For this review, take the finished solid that the model builds, in its own axes (mm). A direction names the side the tool comes from. Give positions to 0.01 mm unless a question says otherwise; leave off trailing zeros. Loops run counter-clockwise (first coordinate to the right, second up) from the corner with the lowest first, then second, coordinate; pieces in that order, holes last. Notation, with made-up numbers: (19.5, 31) - (33.5, 31) arc R8 cw to (33.5, 42) - close; hole circle Ø8 at (6.5, -31). An arc over 180 degrees is marked (long way). Answer in a Markdown table with one row per item.
Autodesk Inventor part; units mm, degrees
ref_plane "YZ Plane" through (0, 0, 0) normal (1, 0, 0) x (0, 1, 0)
ref_plane "XZ Plane" through (0, 0, 0) normal (0, 1, 0) x (-1, 0, 0)
ref_plane "XY Plane" through (0, 0, 0) normal (0, 0, 1) x (1, 0, 0)
sketch "Sketch1" plane through (0, 0, 0) normal (0, 0, 1) x (1, 0, 0)
  line L0 (17, 4.5) -> (17, -4.5)
  line L1 (-17, -4.5) -> (-17, 4.5)
  arc A0 (-8.3666, -4.5) -> (8.3666, -4.5) centre (0, 0) ccw
  arc A1 (8.3666, 4.5) -> (-8.3666, 4.5) centre (0, 0) ccw
  line L2 (-17, 4.5) -> (-8.3666, 4.5)
  line L3 (8.3666, 4.5) -> (17, 4.5)
  line L4 (17, -4.5) -> (8.3666, -4.5)
  line L5 (-8.3666, -4.5) -> (-17, -4.5)
  line L6 (-17, 4.5) -> (17, -4.5) construction
  line L7 (-17, -4.5) -> (17, 4.5) construction
  point P0 (0, 0)
  point P1 (0, 0)
  dimension "d0" = 9
  dimension "d1" = 34
  dimension "d2" = 9.5
  dimension "d3" = 9
  dimension "d4" = 9.5
  dimension "d12" = 4.5
extrude "Extrusion1" add sketch "Sketch1" along normal blind 7
sketch "Sketch2" plane through (17, -4.5, 0) normal (1, 0, 0) x (0, 0, -1)
  arc A0 (-11.5, 9) -> (-11.5, 0) centre (-11.5, 4.5) ccw
  circle A1 centre (-11.5, 4.5) radius 2.25
  line L0 (-7, 9) -> (-11.5, 9)
  line L1 (-11.5, 0) -> (-7, 0)
  line L2 (-7, 0) -> (-7, 9)
  point P0 (0, 4.5)
  point P1 (-7, 0)
  dimension "d7" = 9
  dimension "d8" = 4.5
  dimension "d9" = 9
extrude "Extrusion2" add sketch "Sketch2" against normal blind 4.3
extrude "Extrusion3" add sketch "Sketch2" along normal blind 4.3 from surface at -34
sketch "Sketch3" plane through (-17, -4.5, 0) normal (0, -1, 0) x (1, 0, 0)
  line L0 (0, 6) -> (0, 0)
  line L1 (0, 0) -> (5, 0)
  line L2 (5, 0) -> (0, 6)
  line L3 (29, 0) -> (34, 0)
  line L4 (34, 0) -> (34, 6)
  line L5 (34, 6) -> (29, 0)
  point P0 (17, 0)
  dimension "d15" = 6
  dimension "d16" = 5
  dimension "d17" = 6
  dimension "d18" = 5
extrude "Extrusion4" cut sketch "Sketch3" against normal up to next
sketch "Sketch4" plane through (0, 0, 0) normal (0, 0, -1) x (-1, 0, 0)
  circle A0 centre (0, 0) radius 7.5
  dimension "d21" = 15
extrude "Extrusion5" add sketch "Sketch4" along normal blind 2.5
sketch "Sketch5" plane through (0, 0, 7) normal (0, 0, 1) x (1, 0, 0)
  circle A0 centre (0, 0) radius 7.5
  dimension "d24" = 15
extrude "Extrusion6" cut sketch "Sketch5" against normal blind 4
sketch "Sketch6" plane through (0, 0, -2.5) normal (0, 0, -1) x (-1, 0, 0)
  circle A0 centre (0, 0) radius 5.5
  dimension "d27" = 11
extrude "Extrusion7" cut sketch "Sketch6" against normal blind 4
sketch "Sketch7" plane through (0, 0, 1.5) normal (0, 0, -1) x (-1, 0, 0)
  circle A0 centre (0, 0) radius 5
  dimension "d30" = 10
extrude "Extrusion8" cut sketch "Sketch7" against normal up to next
sketch "Sketch9" plane through (0, 0, 0) normal (1, 0, 0) x (0, 1, 0)
  line L0 (-9.5504, 0) -> (57.3026, 0)
  line L1 (0, -37.6235) -> (0, 29.8791)
  line L2 (9.5, 0) -> (4.5, 0)
  line L3 (9.5, 7) -> (4.5, 7)
  circle A0 centre (30.75, 14.5) radius 1.25
  circle A1 centre (25.75, 13.5) radius 1.25
  line L4 (8.5, 7) -> (9.5, 7)
  line L5 (13.5, 7) -> (13.5, 0) construction
  line L6 (12.4966, 0) -> (8.5, 0)
  line L7 (8.5, 0) -> (8.5, 7)
  line L8 (25.75, 13.5) -> (30.75, 14.5) construction
  line L9 (26.2403, 11.0485) -> (31.2403, 12.0485)
  line L10 (30.2597, 16.9515) -> (25.2597, 15.9515)
  arc A2 (25.2597, 15.9515) -> (26.2403, 11.0485) centre (25.75, 13.5) ccw construction
  arc A3 (31.2403, 12.0485) -> (30.2597, 16.9515) centre (30.75, 14.5) ccw
  arc A4 (25.2597, 15.9515) -> (9.5, 7) centre (49.2826, -44.6916) ccw
  arc A5 (26.2403, 11.0485) -> (14.0842, 0.7836) centre (43.5805, -21.8166) ccw
  arc A6 (12.4966, 0) -> (14.0842, 0.7836) centre (12.4966, 2) ccw
  point P0 (0, 0)
  point P1 (28.25, 14)
  dimension "d133" = 2.5
  dimension "d134" = 30.75
  dimension "d135" = 14.5
  dimension "d136" = 2.5
  dimension "d137" = 13.5
  dimension "d138" = 25.75
  dimension "d139" = 7
  dimension "d140" = 5
  dimension "d141" = 8.5
  dimension "d142" = 5
  dimension "d143" = 65.2279
  dimension "d144" = 37.1592
  dimension "d145" = 2
extrude "Extrusion22" add sketch "Sketch9" along normal mid plane 4
sketch "Sketch19" plane through (0, 0, 0) normal (1, 0, 0) x (0, 1, 0)
  circle A0 centre (25.75, 13.5) radius 1.25
  circle A1 centre (25.75, 13.5) radius 1.25
  circle A2 centre (30.75, 14.5) radius 1.25
  circle A3 centre (30.75, 14.5) radius 1.25
  line L0 (25.75, 13.5) -> (30.75, 14.5) construction
  line L1 (26.2403, 11.0485) -> (31.2403, 12.0485)
  line L2 (30.2597, 16.9515) -> (25.2597, 15.9515)
  arc A4 (25.2597, 15.9515) -> (26.2403, 11.0485) centre (25.75, 13.5) ccw
  arc A5 (31.2403, 12.0485) -> (30.2597, 16.9515) centre (30.75, 14.5) ccw
  point P0 (0, 0)
  point P1 (28.25, 14)
  dimension "d148" = 2.5
  dimension "d149" = 2.5
  dimension "d150" = 5
extrude "Extrusion23" add sketch "Sketch19" along normal blind 3.5
sketch "Sketch20" plane through (0, 0, 0) normal (1, 0, 0) x (0, 1, 0)
  line L0 (0, 4.3) -> (11.7, 4.3)
  line L1 (11.7, 4.3) -> (11.7, 2.7) construction
  line L2 (11.7, 2.7) -> (0, 2.7)
  line L3 (0, 2.7) -> (0, 4.3)
  line L4 (-18.05, 0) -> (41.8, 0)
  line L5 (0, -6.4) -> (0, 20.9)
  line L6 (11.7, 2.7) -> (21.7, 9.2)
  line L7 (11.7, 4.3) -> (20.9843, 10.3348)
  line L8 (20.9843, 10.3348) -> (21.7, 9.2)
  point P0 (0, 0)
  dimension "d153" = 1.6
  dimension "d154" = 11.7
  dimension "d155" = 2.7
  dimension "d156" = 10
  dimension "d157" = 6.5
  dimension "d158" = 1.1348
extrude "Extrusion24" add sketch "Sketch20" along normal mid plane 12
sketch "Sketch21" plane through (0, 0, 7) normal (0, 0, 1) x (1, 0, 0)
  circle A0 centre (0, 0) radius 7.5
  dimension "d161" = 15
extrude "Extrusion25" cut sketch "Sketch5" against normal blind 4
sketch "Sketch22" plane through (0, 0, 1.5) normal (0, 0, -1) x (-1, 0, 0)
  circle A0 centre (0, 0) radius 5
  dimension "d164" = 10
extrude "Extrusion26" cut sketch "Sketch22" against normal through all
sketch "Sketch23" plane through (0, 0, 0) normal (0, 0, 1) x (1, 0, 0)
  line L0 (-6, 21.7) -> (-2, 21.7)
  line L1 (-6, 21.7) -> (-6, 11.7)
  line L2 (-2, 21.7) -> (-6, 21.7)
  line L3 (-6, 7.3655) -> (-6, 11.7)
  line L4 (-6, 21.7) -> (-6, 7.3655)
  arc A0 (-2, 21.7) -> (-6, 7.3655) centre (37.8943, 2.8423) ccw
  line L5 (0, 17.7237) -> (0, 15.5632) construction
  line L6 (6, 21.7) -> (2, 21.7)
  line L7 (6, 21.7) -> (6, 11.7)
  line L8 (6, 7.3655) -> (6, 11.7)
  arc A1 (6, 7.3655) -> (2, 21.7) centre (-37.8943, 2.8423) ccw
  point P0 (0, 0)
extrude "Extrusion27" cut sketch "Sketch23" along normal through all
properties part number "RCT-P006_steering_knuckle"
1. We need section C-C, the plane x = -11. Give the boundary of the cut face in (y, z).
Values:
| item | result |
|---|---|
| outline | (-4.5, 0) - (4.5, 0) - (4.5, 7) - (-4.5, 7) - close |
2. Mouldability with a two-part tool opening along Z and no side actions: class faces 5 (the face through (-15, 0, 16)), 6 (the face through (-0.03, 19.52, 6.5)), 7 (the face through (0.712, 31.422, 13.446)) as released by +Z, released by -Z, zero draft, split by the parting line, or undercut.
Values:
| item | result |
|---|---|
| face 5 | released by +Z |
| face 6 | released by -Z |
| face 7 | undercut |
3. Clearance check with flat-ended pins moving along their axes: pin 1 (8 mm diameter, centred on x = 6, y = 28, fed in from -Z); pin 2 (6 mm diameter, centred on y = 17, z = 14.5, fed in from +X); pin 3 (2 mm diameter, centred on y = 25.75, z = 13.5, fed in from +X); pin 4 (2 mm diameter, centred on x = 12, z = 7.5, fed in from -Y). State where each tip first meets the part, or that it passes through.
Values:
| item | result |
|---|---|
| pin 1 | stops at z = 11 |
| pin 2 | stops at x = 2 |
| pin 3 | passes through |
| pin 4 | stops at y = -4.5 |
4. We need section B-B, the plane y = 30.75. Give the boundary of the cut face in (x, z), and give its area (3 significant figures).
Values:
| item | result |
|---|---|
| outline | (-2, 11.95) - (3.5, 11.95) - (3.5, 13.25) - (-2, 13.25) - close; (-2, 15.75) - (3.5, 15.75) - (3.5, 17) - (-2, 17) - close |
| area | 14.0 mm^2 |
5. Wall thickness on line 1 (Y direction, x = -15.15, z = 11.5); line 2 (X direction, y = 3.5, z = 14); line 3 (Y direction, x = -4.5, z = 2.75): over which ranges is each line inside the solid? List them lowest first. Write a range as [from, to].
Values:
| item | result |
|---|---|
| line 1 | y = [-4.5, -2.25], [2.25, 4.5] |
| line 2 | x = [-17, -12.7], [12.7, 17] |
| line 3 | y = [-8.37, -2.18], [2.18, 11.78] |
6. We need section A-A, the plane y = 0. Count the separate pieces of the cut face and the enclosed holes in it, and give its area (3 significant figures).
Values:
| item | result |
|---|---|
| separate pieces | 4 |
| enclosed holes | 0 |
| area | 165 mm^2 |
7. We need section D-D, the plane z = -0.5. Give the boundary of the cut face in (x, y), and give its area (3 significant figures).
Values:
| item | result |
|---|---|
| outline | circle Ø15 at (0, 0); hole circle Ø11 at (0, 0) |
| area | 81.7 mm^2 |
8. For faces 1 (the face through (7.493, -0.33, -1.232)), 2 (the face through (-7.493, 0.33, 5.028)), 3 (the face through (2, 16, 8)), 4 (the face through (-3.32, 15.519, 5.182)), list the 3-axis set-ups (+Z, -Z, +X, -X, +Y, -Y) from which the entire face can be reached by the end or side of a thin tool; tool diameter is ignored.
Values:
| item | result |
|---|---|
| face 1 | -Z |
| face 2 | +Z |
| face 3 | +X |
| face 4 | -Z, -X, +Y |
